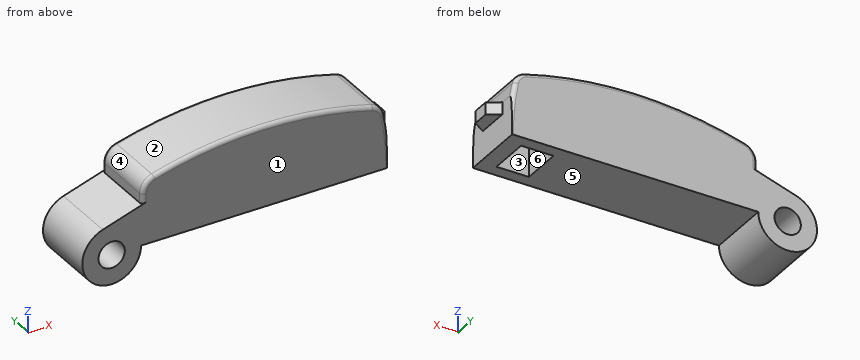
from build123d import *

# Parameters (mm, degrees)
SKETCH1_R           = 1.625
BOSS_EXTRUDE1_DEPTH = 4
BOSS_EXTRUDE2_DEPTH = 1.5
FILLET1_R           = 0.5
SKETCH4_W           = 4
SKETCH4_H           = 5
CUT_EXTRUDE1_DEPTH  = 4


with BuildPart() as part:
    # Sketch1 → Boss-Extrude1 (new, symmetric)
    with BuildSketch(Plane(origin=(0, 0, 0), x_dir=(1, 0, 0), z_dir=(0, 1, 0))):
        with BuildLine():
            Line((34, 0), (3.625, 0))
            ThreePointArc((3.625, 0), (-2.138914072, 2.926716862), (-1.100887775, -3.453790831))
            Line((-1.100887775, -3.453790831), (3.75, -5))
            Line((3.75, -5), (3.75, -6.203874108))
            ThreePointArc((3.75, -6.203874108), (4.15563796, -7.411354826), (5.208009684, -8.12903553))
            ThreePointArc((5.208009684, -8.12903553), (18.757767579, -10), (32.307525473, -8.12903553))
            ThreePointArc((32.307525473, -8.12903553), (33.236223507, -7.559261794), (33.728449863, -6.587235373))
            ThreePointArc((33.728449863, -6.587235373), (33.873522982, -5.795208431), (34, -5))
            Line((34, -5), (34, 0))
        make_face()
        Circle(SKETCH1_R, mode=Mode.SUBTRACT)
    extrude(amount=BOSS_EXTRUDE1_DEPTH, both=True)

    # Sketch3 → Boss-Extrude2 (add)
    with BuildSketch(Plane(origin=(0, 0, 5), x_dir=(-1, 0, 0), z_dir=(0, 0, -1))):
        Polygon((-34, -2), (-35.5, -1), (-35.5, 1), (-34, 2), align=None)
    extrude(amount=BOSS_EXTRUDE2_DEPTH)

    # Fillet1
    fillet1_edges = [part.edges().sort_by_distance(p)[0] for p in [
        (3.75, 4, 5.601937054),
        (4.15563796, 4, 7.411354826),
        (33.873522982, 4, 5.795208431),
        (33.236223507, 4, 7.559261794),
        (3.75, -4, 5.601937054),
        (4.15563796, -4, 7.411354826),
        (33.873522982, -4, 5.795208431),
        (33.236223507, -4, 7.559261794),
        (18.757767579, 4, 10),
        (18.757767579, -4, 10),
    ]]
    fillet(fillet1_edges, radius=FILLET1_R)

    # Sketch4 → Cut-Extrude1 (cut)
    with BuildSketch(Plane(origin=(0, 0, 0), x_dir=(-1, 0, 0), z_dir=(0, 0, -1))):
        with Locations((-30, 0)):
            Rectangle(SKETCH4_W, SKETCH4_H)
    extrude(amount=-CUT_EXTRUDE1_DEPTH, mode=Mode.SUBTRACT)


solid = part.part
For this review, take the finished solid that the model builds, in its own axes (mm). Face numbers are marked on the shaded views. A direction names the side the tool comes from. Give positions to 0.01 mm unless a question says otherwise; leave off trailing zeros. Write each loop counter-clockwise with the first axis right and the second up, starting at its lowest first coordinate (ties: lowest second). Pieces come first, ordered by that corner, then holes. Notation, with made-up numbers: (38.25, 85) -> (60.25, 85) arc R11 ccw to (60.25, 105) -> close; hole circle Ø3 at (-39, 78). An arc over 180 degrees is marked (long way). Use CSV: the item, a comma, the result in double quotes.
Q1. Tool access review of the marked faces 4, 5 and 6: name each direction out of +Z, -Z, +X, -X, +Y, -Y from which nothing blocks a thin tool from reaching the whole face with its end or side.
Conclusion:
face 4,"+Z, -X, +Y, -Y"
face 5,"-Z, +X, +Y, -Y"
face 6,"-Z"
Q2. Take a section at A-A, the plane x = 0. Write out the cut boundary in (y, z) (3 decimals).
Conclusion:
outline,"(-4, -3.625) -> (4, -3.625) -> (4, -1.625) -> (-4, -1.625) -> close; (-4, 1.625) -> (4, 1.625) -> (4, 3.805) -> (-4, 3.805) -> close"
Q3. Mouldability with a two-part tool opening along Y and no side actions: class the marked faces 1, 2 and 3 as pulls with the +Y half, pulls with the -Y half, needs draft (parallel to the pull), parting line crosses it, or undercut.
Conclusion:
face 1,"pulls with the -Y half"
face 2,"needs draft"
face 3,"undercut"
Q4. For P1, Ø2, axis at x = 29.5, y = -0.5, coming from the -Z side; P2, Ø2.5, axis at x = 11.5, y = 0.5, coming from the -Z side; P3, Ø4, axis at x = 1, y = 1, coming from the +Z side, all flat-tipped, find the tip position at first contact; note any pin that passes through.
Conclusion:
P1,"z = 4"
P2,"z = 0"
P3,"z = 4.76"
Q5. To check wall thickness, follow probe 1 along X at (y, z) = (-1.75, 0.25); probe 2 along X at (y, z) = (-1.5, 2); probe 3 along X at (y, z) = (-1, 2.25). State the ranges of each line that lie inside material, in increasing order. Write a range as [from, to].
Conclusion:
probe 1,"[-3.62, -1.61], [1.61, 28], [32, 34]"
probe 2,"[-3.02, 28], [32, 34]"
probe 3,"[-2.84, 28], [32, 34]"
Q6. Take a section at B-B, the plane z = -0.5. Write out the cut boundary in (x, y).
Conclusion:
outline,"(-3.59, -4) -> (-1.55, -4) -> (-1.55, 4) -> (-3.59, 4) -> close; (1.55, -4) -> (3.59, -4) -> (3.59, 4) -> (1.55, 4) -> close"
